Geometry: final body of the model. Coordinates: model frame, mm. Round coordinates to 2 decimals unless told otherwise and drop trailing zeros. Loops run counter-clockwise (first coordinate to the right, second up) from the corner with the lowest first, then second, coordinate; pieces in that order, holes last. Notation, with made-up numbers: M 51.5,74.25 L 108.5,74.25 A14 cw 108.5,78.25 Z; hole C 12,-16 d1. An arc over 180 degrees is marked long. Answer as a JSON object with one key per item and string values.
from build123d import *

# Parameters (mm, degrees)
F0_W     = 1295.4
F0_H     = 584.2
F1_DEPTH = 19.05
F3_DEPTH = 25.4
F4_R     = 50.8
F5_W     = 82.55
F5_H     = 9.525
F6_DEPTH = 1295.401


with BuildPart() as f1:
    # F0 (on Top) → F1 (new body)
    with BuildSketch(Plane.XY):
        Rectangle(F0_W, F0_H)
    extrude(amount=F1_DEPTH)

    # F2 (on face) → F3 (cut)
    with BuildSketch(Plane.XY.offset(19.05)):
        with BuildLine():
            Line((-159.4836327272, 33.408662691), (-304.8, -292.1))
            Line((-304.8, -292.1), (520.7, -292.1))
            Line((520.7, -292.1), (375.3836327272, 33.408662691))
            ThreePointArc((375.3836327272, 33.408662691), (356.6425656273, 55.3183063055), (328.9962282994, 63.5))
            Line((328.9962282994, 63.5), (-113.0962282994, 63.5))
            ThreePointArc((-113.0962282994, 63.5), (-140.7425656273, 55.3183063055), (-159.4836327272, 33.408662691))
        make_face()
    extrude(amount=-F3_DEPTH, mode=Mode.SUBTRACT)

    # F4
    f4_edges = [f1.edges().sort_by_distance(p)[0] for p in [
        (-304.8, -292.1, 9.525),
        (520.7, -292.1, 9.525),
        (647.7, -292.1, 9.525),
        (-647.7, -292.1, 9.525),
    ]]
    fillet(f4_edges, radius=F4_R)

    # F5 (on face) → F6 (cut, through all)
    with BuildSketch(Plane.YZ.offset(647.7)):
        with Locations((250.825, 4.7625)):
            Rectangle(F5_W, F5_H)
    extrude(amount=-F6_DEPTH, mode=Mode.SUBTRACT)


solid = f1.part
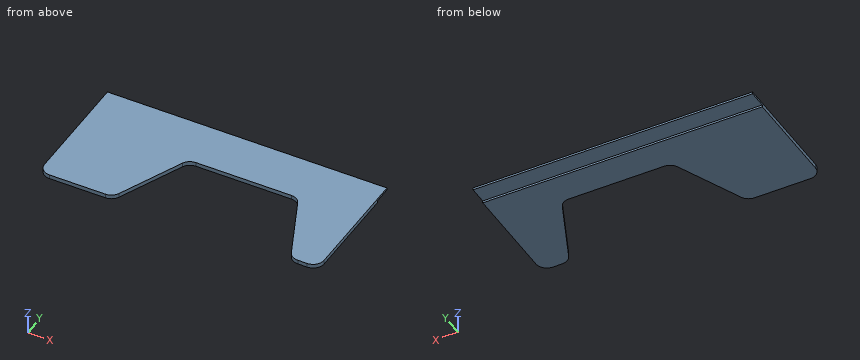
1) Section query B-B (y = -63). Return the cut outline in (x, z), and give its area (3 significant figures).
Results:
{"outline": "M -647.7,0 L -202.52,0 L -202.52,19.05 L -647.7,19.05 Z; M 418.42,0 L 647.7,0 L 647.7,19.05 L 418.42,19.05 Z", "area": "12,800 mm2"}
2) Ray query, line 1 (Z direction, x = 96.5, y = 262.5) (3 decimals); line 2 (Y direction, x = -354, z = 6); line 3 (X direction, y = -14, z = 1.25). Return the intervals inside material, ascending.
Results:
{"line 1": "9.525 to 19.05", "line 2": "-292.1 to 209.55", "line 3": "-647.7 to -180.65, 396.55 to 647.7"}
3) Section query C-C (x = 180.5). Return the cut outline in (y, z) (3 decimals), and give its area (3 significant figures).
Results:
{"outline": "M 63.5,0 L 209.55,0 L 209.55,9.525 L 292.1,9.525 L 292.1,19.05 L 63.5,19.05 Z", "area": "3,570 mm2"}
4) Section query A-A (z = 16). Return the cut outline in (x, y), and give its area (3 significant figures).
Results:
{"outline": "M -647.7,-241.3 A50.8 ccw -596.9,-292.1 L -337.75,-292.1 A50.8 ccw -291.37,-262.01 L -159.48,33.41 A50.8 cw -113.1,63.5 L 329,63.5 A50.8 cw 375.38,33.41 L 507.27,-262.01 A50.8 ccw 553.65,-292.1 L 596.9,-292.1 A50.8 ccw 647.7,-241.3 L 647.7,292.1 L -647.7,292.1 Z", "area": "519,000 mm2"}
5) Section query D-D (y = -156.5). Return the cut outline in (x, z), and give its area (3 significant figures).
Results:
{"outline": "M -647.7,0 L -244.26,0 L -244.26,19.05 L -647.7,19.05 Z; M 460.16,0 L 647.7,0 L 647.7,19.05 L 460.16,19.05 Z", "area": "11,300 mm2"}
6) Pin query (flat end, axial travel): P1, Ø8, axis at x = 225, z = 11.5, coming from the -Y side; P2, Ø3, axis at x = 33.5, z = 3, coming from the +Y side; P3, Ø25, axis at x = 183.5, y = 240.5, coming from the -Z side (3 decimals). Return the tip coordinate at first contact, or that it passes through.
Results:
{"P1": "y = 63.5", "P2": "y = 209.55", "P3": "z = 9.525"}
